```python
from build123d import *

# Parameters (mm, degrees)
F0_W     = 24
F0_H     = 45
F0_R     = 5.1
F1_DEPTH = 15
F2_R     = 5
F3_R     = 1.5
F4_DEPTH = 24


with BuildPart() as f1:
    # F0 (on Right) → F1 (new body)
    with BuildSketch(Plane.YZ):
        with Locations((0, -22.5)):
            Rectangle(F0_W, F0_H)
        with Locations((0, -9)):
            Circle(F0_R, mode=Mode.SUBTRACT)
    extrude(amount=F1_DEPTH)

    # F2
    f2_edges = [f1.edges().sort_by_distance(p)[0] for p in [
        (7.5, 12, 0),
        (7.5, -12, 0),
    ]]
    fillet(f2_edges, radius=F2_R)

    # F3 (on face) → F4 (cut, through all)
    with BuildSketch(Plane.XZ.offset(12)):
        with Locations((7.5, -9)):
            Circle(F3_R)
    extrude(amount=-F4_DEPTH, mode=Mode.SUBTRACT)


solid = f1.part
```
Design review of the part built by this model. Coordinates are the model's own, in mm. Give positions to 0.01 mm unless a question says otherwise; leave off trailing zeros. Order: outer loops, then holes, each group sorted by start corner. A loop starts at its lowest first (then second) coordinate and runs counter-clockwise, first axis right, second up. Notation, with made-up numbers: M 32.5,-23.5 L 75.5,-23.5 A22 cw 75.5,-15.5 Z; hole C 17.25,-3 d9. An arc over 180 degrees is marked long. One line per question, with ' | ' between items. Start each with the question number.
Q1. We need section A-A (z = -9). Write out the cut boundary in (x, y), plus the area to 3 significant figures.
Q2. For pin 1 Ø9 at (y, z) = (0, -9) entering from +X, flat-tipped, find the tip position at first contact; note if it passes through.
Q3. We need section B-B (y = 0). Write out the cut boundary in (x, z).
Q4. We need section C-C (x = 10). Write out the cut boundary in (y, z).
Q5. The part is to be moulded in two halves that separate along Y. For faces 1 (the face through (7.395, 4.711, -10.953)), 2 (the face through (6.3, 8.4, -9.9)), 3 (the face through (7, 12, -25)), 4 (the face through (8, -11, -2)), say which applies: +Y half, -Y half, draft (parallel to the pull), parting line (faces both ways), or undercut.
Q6. We need section D-D (x = 7.5). Write out the cut boundary in (y, z).
Q7. For L1, parallel to X at y = 9.25, z = -9; L2, parallel to Y at x = 11.5, z = -9; L3, parallel to Z at x = 11, y = -0.25, list the stretches that pass through material, from the lowest coordinate up. Write a range as [from, to].
Returned:
1) outline: M 0,-12 L 6,-12 L 6,-5.1 L 0,-5.1 Z; M 0,5.1 L 6,5.1 L 6,12 L 0,12 Z; M 9,-12 L 15,-12 L 15,-5.1 L 9,-5.1 Z; M 9,5.1 L 15,5.1 L 15,12 L 9,12 Z | area: 166 mm2
2) pin 1: through
3) outline: M 0,-45 L 15,-45 L 15,-14.1 L 0,-14.1 Z; M 0,-3.9 L 15,-3.9 L 15,0 L 0,0 Z
4) outline: M -12,-45 L 12,-45 L 12,-5 A5 ccw 7,0 L -7,0 A5 ccw -12,-5 Z; hole C 0,-9 d10.2
5) face 1: undercut | face 2: draft | face 3: +Y half | face 4: -Y half
6) outline: M -12,-45 L 12,-45 L 12,-10.5 L 4.87,-10.5 A5.1 cw -4.87,-10.5 L -12,-10.5 Z; M -12,-7.5 L -4.87,-7.5 A5.1 cw 4.87,-7.5 L 12,-7.5 L 12,-5 A5 ccw 7,0 L -7,0 A5 ccw -12,-5 Z
7) L1: [0, 6], [9, 15] | L2: [-12, -5.1], [5.1, 12] | L3: [-45, -14.09], [-3.91, 0]
